from build123d import *

# Parameters (mm, degrees)
SKETCH_1_R      = 2
EXTRUDE_1_DEPTH = 1
FILLET_1_R      = 2
FILLET_2_R      = 0.5
SKETCH_3_R      = 2
SKETCH_3_R_2    = 1
EXTRUDE_2_DEPTH = 5.5


with BuildPart() as part:
    # 草图1 → 凸台-拉伸1 (new body)
    with BuildSketch(Plane(origin=(0, 0, 0), x_dir=(1, 0, 0), z_dir=(0, 1, 0))):
        Polygon((-12.5, 1), (-5.5, 1), (-5.5, 0), (5.5, 0), (5.5, 1), (12.5, 1), (12.5, 8), (-12.5, 8), align=None)
        with Locations(Location((8.5, 4.5, 0), (0, 0, 270))):
            Circle(SKETCH_1_R, mode=Mode.SUBTRACT)
        with Locations(Location((-8.5, 4.5, 0), (0, 0, 270))):
            Circle(SKETCH_1_R, mode=Mode.SUBTRACT)
    extrude(amount=EXTRUDE_1_DEPTH)

    # 圆角1
    fillet_1_edges = [part.edges().sort_by_distance(p)[0] for p in [
        (-12.5, 0.5, -8),
        (12.5, 0.5, -8),
    ]]
    fillet(fillet_1_edges, radius=FILLET_1_R)

    # 圆角2
    fillet_2_edges = [part.edges().sort_by_distance(p)[0] for p in [
        (5.5, 0.5, -1),
        (-5.5, 0.5, -1),
    ]]
    fillet(fillet_2_edges, radius=FILLET_2_R)

    # 草图3 → 凸台-拉伸2 (add, symmetric)
    with BuildSketch(Plane(origin=(0, 0, 0), x_dir=(0, 0, -1), z_dir=(1, 0, 0))):
        with Locations((-1.5, 1.322875656)):
            Circle(SKETCH_3_R)
        with Locations((-1.5, 1.322875656)):
            Circle(SKETCH_3_R_2, mode=Mode.SUBTRACT)
    extrude(amount=EXTRUDE_2_DEPTH, both=True)


solid = part.part
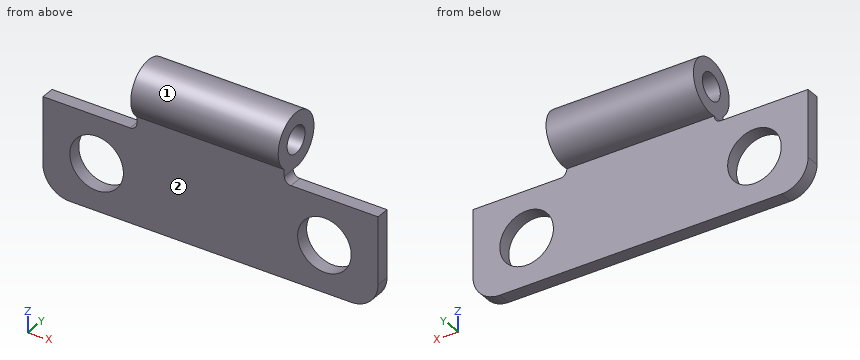
Verification items for the finished model (mm, model axes). Face numbers are marked on the shaded views. A direction names the side the tool comes from. Coordinates: 2 decimals unless noted, no trailing zeros. Write each loop counter-clockwise with the first axis right and the second up, starting at its lowest first coordinate (ties: lowest second). Pieces come first, ordered by that corner, then holes. Notation, with made-up numbers: (9.25, 10) -> (35.25, 10) arc R16 cw to (35.25, 35) -> close; hole circle Ø11 at (70, 13.5). An arc over 180 degrees is marked (long way). One line per item, written item: value. Start each with the question number.
Q1. Thickness scan on L1, parallel to X at y = 0.45, z = -4.5; L2, parallel to Y at x = 1.25, z = 1.5; L3, parallel to Y at x = 6, z = -5.5. Record the ranges inside material, lowest first. Write a range as from..to.
Q2. Cross-section at A-A on z = 1.5. Enter the section's corners in (x, y), and give its area (3 significant figures).
Q3. Cross-section at C-C on z = -6.25. Enter the section's corners in (x, y).
Q4. Cross-section at D-D on x = -1.5. Enter the section's corners in (y, z).
Q5. Go/stop test with flat-tipped pins: P1, Ø1.2, axis at y = 1, z = 2, coming from the -X side; P2, Ø4.5, axis at x = -8.5, z = -4.5, coming from the +Y side; P3, Ø2, axis at x = 7.5, y = -0.5, coming from the +Z side; P4, Ø1.2, axis at y = 1.32, z = 1.5, coming from the -X side. Record where each tip stops, or that it passes through.
Q6. Cross-section at B-B on x = -8.5. Enter the section's corners in (y, z), and give its area (3 significant figures).
Q7. Access from +Z, -Z, +X, -X, +Y, -Y to the whole of each face (thin tool, end or side, straight path). Record for the marked faces 1 and 2.
Checked values:
1. L1: x = -12.5..-10.5, -6.5..6.5, 10.5..12.5
1. L2: y = -0.68..0.32, 2.32..3.32
1. L3: y = 0..1
2. outline: (-5.5, -0.68) -> (5.5, -0.68) -> (5.5, 0.32) -> (-5.5, 0.32) -> close; (-5.5, 2.32) -> (5.5, 2.32) -> (5.5, 3.32) -> (-5.5, 3.32) -> close
2. area: 22.0 mm²
3. outline: (-12.48, 0) -> (-9.47, 0) -> (-9.47, 1) -> (-12.48, 1) -> close; (-7.53, 0) -> (7.53, 0) -> (7.53, 1) -> (-7.53, 1) -> close; (9.47, 0) -> (12.48, 0) -> (12.48, 1) -> (9.47, 1) -> close
4. outline: (0, -8) -> (1, -8) -> (1, -0.47) arc R2 ccw (long way) to (0, 0) -> close; hole circle Ø2 at (1.32, 1.5)
5. P1: stops at x = -5.5
5. P2: stops at y = 1
5. P3: stops at z = -1
5. P4: passes through
6. outline: (0, -8) -> (1, -8) -> (1, -6.5) -> (0, -6.5) -> close; (0, -2.5) -> (1, -2.5) -> (1, -1) -> (0, -1) -> close
6. area: 3.00 mm²
7. face 1: +X, -X
7. face 2: -Z, +X, -X, -Y
